For this review, take the finished solid that the model builds, in its own axes (mm). A direction names the side the tool comes from. Give positions to 0.01 mm unless a question says otherwise; leave off trailing zeros. Order: outer loops, then holes, each group sorted by start corner. A loop starts at its lowest first (then second) coordinate and runs counter-clockwise, first axis right, second up.
from build123d import *

# Parameters (mm, degrees)
SKICA1_W                = 97.8
SKICA1_H                = 60.8
SKICA1_W_2              = 11.8
SKICA1_H_2              = 14.8
SKICA1_W_3              = 5.4
SKICA1_H_3              = 5.4
P_IDAT_VYSUNUT_M1_DEPTH = 2.6
SKICA1_3_W              = 102
SKICA1_3_H              = 65
SKICA1_3_W_2            = 97.8
SKICA1_3_H_2            = 60.8
P_IDAT_VYSUNUT_M2_DEPTH = 1
SKICA1_5_W              = 11.8
SKICA1_5_H              = 14.8
SKICA1_5_W_2            = 5.4
SKICA1_5_H_2            = 5.4
P_IDAT_VYSUNUT_M3_DEPTH = 0.2
ZAOBLIT1_R              = 3
ZAOBLIT2_R              = 3
SKICA1_6_W              = 97.8
SKICA1_6_H              = 60.8
SKICA1_6_W_2            = 93.8
SKICA1_6_H_2            = 56.8
P_IDAT_VYSUNUT_M4_DEPTH = 5.6
ZAOBLIT4_R              = 3
ZAOBLIT5_R              = 3


with BuildPart() as part:
    # Skica1 → Přidat vysunutím1 (new body)
    with BuildSketch(Plane.XY):
        with Locations((51, 32.5)):
            Rectangle(SKICA1_W, SKICA1_H)
        with Locations((15, 16.5)):
            Rectangle(SKICA1_W_2, SKICA1_H_2, mode=Mode.SUBTRACT)
        with Locations((36.8, 16.5)):
            Rectangle(SKICA1_W_2, SKICA1_H_2, mode=Mode.SUBTRACT)
        with Locations((58.6, 16.5)):
            Rectangle(SKICA1_W_2, SKICA1_H_2, mode=Mode.SUBTRACT)
        with Locations((82.1, 16.5)):
            Rectangle(SKICA1_W_3, SKICA1_H_3, mode=Mode.SUBTRACT)
    extrude(amount=P_IDAT_VYSUNUT_M1_DEPTH)

    # Skica1<3> → Přidat vysunutím2 (add)
    with BuildSketch(Plane.XY):
        with Locations((51, 32.5)):
            Rectangle(SKICA1_3_W, SKICA1_3_H)
        with Locations((51, 32.5)):
            Rectangle(SKICA1_3_W_2, SKICA1_3_H_2, mode=Mode.SUBTRACT)
    extrude(amount=P_IDAT_VYSUNUT_M2_DEPTH)

    # Skica1<5> → Přidat vysunutím3 (add)
    with BuildSketch(Plane.XY):
        with Locations((58.6, 16.5)):
            Rectangle(SKICA1_5_W, SKICA1_5_H)
        with Locations((15, 16.5)):
            Rectangle(SKICA1_5_W, SKICA1_5_H)
        with Locations((36.8, 16.5)):
            Rectangle(SKICA1_5_W, SKICA1_5_H)
        with Locations((82.1, 16.5)):
            Rectangle(SKICA1_5_W_2, SKICA1_5_H_2)
    extrude(amount=P_IDAT_VYSUNUT_M3_DEPTH)

    # Zaoblit1
    zaoblit1_edges = [part.edges().sort_by_distance(p)[0] for p in [
        (0, 0, 0.5),
        (102, 0, 0.5),
        (102, 65, 0.5),
        (0, 65, 0.5),
    ]]
    fillet(zaoblit1_edges, radius=ZAOBLIT1_R)

    # Zaoblit2
    zaoblit2_edges = [part.edges().sort_by_distance(p)[0] for p in [
        (99.9, 2.1, 1.8),
        (99.9, 62.9, 1.8),
        (2.1, 62.9, 1.8),
        (2.1, 2.1, 1.8),
    ]]
    fillet(zaoblit2_edges, radius=ZAOBLIT2_R)

    # Skica1<6> → Přidat vysunutím4 (add)
    with BuildSketch(Plane.XY):
        with Locations((51, 32.5)):
            Rectangle(SKICA1_6_W, SKICA1_6_H)
        with Locations((51, 32.5)):
            Rectangle(SKICA1_6_W_2, SKICA1_6_H_2, mode=Mode.SUBTRACT)
    extrude(amount=P_IDAT_VYSUNUT_M4_DEPTH)

    # Zaoblit4
    zaoblit4_edges = [part.edges().sort_by_distance(p)[0] for p in [
        (2.1, 62.9, 3.3),
        (99.9, 2.1, 3.3),
        (2.1, 2.1, 3.3),
        (99.9, 62.9, 3.3),
    ]]
    fillet(zaoblit4_edges, radius=ZAOBLIT4_R)

    # Zaoblit5
    zaoblit5_edges = [part.edges().sort_by_distance(p)[0] for p in [
        (4.1, 60.9, 4.1),
        (97.9, 60.9, 4.1),
        (97.9, 4.1, 4.1),
        (4.1, 4.1, 4.1),
    ]]
    fillet(zaoblit5_edges, radius=ZAOBLIT5_R)


solid = part.part
1) Clearance check with flat-ended pins moving along their axes: pin 1 (1 mm diameter, centred on x = 17.5, y = 28.5, fed in from +Z); pin 2 (1.2 mm diameter, centred on x = 38, z = 2, fed in from +Y); pin 3 (3.5 mm diameter, centred on x = 39, y = 13, fed in from +Z). State where each tip first meets the part, or that it passes through.
Answer sheet:
pin 1: stops at z = 2.6
pin 2: stops at y = 62.9
pin 3: stops at z = 0.2
2) We need section D-D on x = 73. Give the boundary of the cut face in (y, z).
Answer sheet:
outline: (0, 0) - (65, 0) - (65, 1) - (62.9, 1) - (62.9, 5.6) - (60.9, 5.6) - (60.9, 2.6) - (4.1, 2.6) - (4.1, 5.6) - (2.1, 5.6) - (2.1, 1) - (0, 1) - close
3) To check wall thickness, follow line 1 (X direction, y = 12, z = 2.2); line 2 (X direction, y = 15, z = 1.6); line 3 (Y direction, x = 41, z = 4.1). State the ranges of each line that lie inside material, in increasing order.
Answer sheet:
line 1: x = 2.1 to 9.1, 20.9 to 30.9, 42.7 to 52.7, 64.5 to 99.9
line 2: x = 2.1 to 9.1, 20.9 to 30.9, 42.7 to 52.7, 64.5 to 79.4, 84.8 to 99.9
line 3: y = 2.1 to 4.1, 60.9 to 62.9
4) We need section A-A on z = 3.5. Give the boundary of the cut face in (x, y), then the cut area to 3 significant figures.
Answer sheet:
outline: (2.1, 5.1) arc R3 ccw to (5.1, 2.1) - (96.9, 2.1) arc R3 ccw to (99.9, 5.1) - (99.9, 59.9) arc R3 ccw to (96.9, 62.9) - (5.1, 62.9) arc R3 ccw to (2.1, 59.9) - close; hole (4.1, 7.1) arc R3 ccw to (7.1, 4.1) - (94.9, 4.1) arc R3 ccw to (97.9, 7.1) - (97.9, 57.9) arc R3 ccw to (94.9, 60.9) - (7.1, 60.9) arc R3 ccw to (4.1, 57.9) - close
area: 618 mm2
5) We need section C-C on x = 36.5. Give the boundary of the cut face in (y, z), then the cut area to 3 significant figures.
Answer sheet:
outline: (0, 0) - (65, 0) - (65, 1) - (62.9, 1) - (62.9, 5.6) - (60.9, 5.6) - (60.9, 2.6) - (23.9, 2.6) - (23.9, 0.2) - (9.1, 0.2) - (9.1, 2.6) - (4.1, 2.6) - (4.1, 5.6) - (2.1, 5.6) - (2.1, 1) - (0, 1) - close
area: 139 mm2
6) Draft analysis for pull direction Y (two halves, no side actions). For faces 6 (the face through (37, 17, 0.2)), 7 (the face through (101.14, 64.1, 0.51)), 8 (the face through (50, 33, 0)), state which applies: +Y half, -Y half, draft (parallel to the pull), parting line (faces both ways), or undercut.
Answer sheet:
face 6: undercut
face 7: +Y half
face 8: draft
7) Tool access review of faces 1 (the face through (2.1, 32, 3)), 2 (the face through (59, 23.9, 1)), 3 (the face through (99, 2.96, 3.33)), 4 (the face through (99.9, 32, 3)), 5 (the face through (50, 62.9, 3)): name each direction out of +Z, -Z, +X, -X, +Y, -Y from which nothing blocks a thin tool from reaching the whole face with its end or side.
Answer sheet:
face 1: +Z, -X, +Y, -Y
face 2: +Z
face 3: +Z, +X, -Y
face 4: +Z, +X, +Y, -Y
face 5: +Z, +X, -X, +Y
8) We need section B-B on y = 47. Give the boundary of the cut face in (x, z).
Answer sheet:
outline: (0, 0) - (102, 0) - (102, 1) - (99.9, 1) - (99.9, 5.6) - (97.9, 5.6) - (97.9, 2.6) - (4.1, 2.6) - (4.1, 5.6) - (2.1, 5.6) - (2.1, 1) - (0, 1) - close
